from build123d import *

# Parameters (mm, degrees)
F1_DEPTH = 15
F4_D     = 4.1
F4_DEPTH = 7
F5_D     = 6.1
F5_DEPTH = 7


with BuildPart() as f1:
    # F0 (on Top) → F1 (new body)
    with BuildSketch(Plane.XY):
        Polygon((-8.678603, -7.1), (-8.678603, -5.1), (-10.678603, -7.1), (-10.678603, -13.5), (16.421397, -13.5), (16.421397, 13), (11.421397, 13), (11.421397, -7.1), (6.971397, -7.1), (6.971397, -10.4), (-4.228603, -10.4), (-4.228603, -7.1), align=None)
    extrude(amount=F1_DEPTH)

    # F4
    with Locations(Plane.YZ.offset(16.421397)):
        with Locations((3, 7.5)):
            Hole(F4_D / 2, depth=F4_DEPTH)

    # F5
    with Locations(Plane.XZ.offset(13.5)):
        with Locations((1.371397, 7.5)):
            Hole(F5_D / 2, depth=F5_DEPTH)


solid = f1.part
Could you check a few things on this model? Use its own coordinates, in mm. A direction names the side the tool comes from. Give positions to 0.01 mm unless a question says otherwise; leave off trailing zeros. Order: outer loops, then holes, each group sorted by start corner. A loop starts at its lowest first (then second) coordinate and runs counter-clockwise, first axis right, second up.
Item 1: I need wall thicknesses on line 1 (X direction, y = -7.75, z = 1); line 2 (Z direction, x = 15.05, y = 3); line 3 (Y direction, x = 7.75, z = 1). Which ranges of each line are inside material? Lowest first, please.
Item 2: If we section it at D-D, the plane z = 13: Write out the boundary of the cut face in (x, y).
Item 3: If we section it at B-B, the plane z = 7.5: Write out the boundary of the cut face in (x, y).
Item 4: I'm going to push flat-ended pins straight in: pin 1 (3.5 mm diameter, centred on y = 3, z = 7.5, fed in from -X); pin 2 (3.5 mm diameter, centred on x = 2.5, z = 6, fed in from +Y); pin 3 (1.3 mm diameter, centred on x = -6, z = 11, fed in from +Y). Where does each tip first touch, or does it pass through?
Item 5: If we section it at C-C, the plane x = 12.5: Write out the boundary of the cut face in (y, z), plus the area to 3 significant figures.
Item 6: If we mould it in two halves opening along Y, with no side actions, what happens to faces 3 (the face through (13.89, 1.11, 6.71)), 4 (the face through (-9.665, -6.086, 7.395)), 5 (the face through (-8.679, -6, 7))? For each: pulls with the +Y half, pulls with the -Y half, needs draft (parallel to the pull), parting line crosses it, or undercut.
Item 7: For faces 1 (the face through (-4.229, -9, 7)), 2 (the face through (16.421, 0, 7)), which set-ups out of +Z, -Z, +X, -X, +Y, -Y let a thin tool reach every point of the face, with its end or its side?
Item 8: If we section it at A-A, the plane y = 3: Write out the boundary of the cut face in (x, z), plus the area to 3 significant figures.
Values:
1. line 1: x = -10.68 to -4.23, 6.97 to 16.42
1. line 2: z = 0 to 5.45, 9.55 to 15
1. line 3: y = -13.5 to -7.1
2. outline: (-10.68, -13.5) - (16.42, -13.5) - (16.42, 13) - (11.42, 13) - (11.42, -7.1) - (6.97, -7.1) - (6.97, -10.4) - (-4.23, -10.4) - (-4.23, -7.1) - (-8.68, -7.1) - (-8.68, -5.1) - (-10.68, -7.1) - close
3. outline: (-10.68, -13.5) - (-1.68, -13.5) - (-1.68, -10.4) - (-4.23, -10.4) - (-4.23, -7.1) - (-8.68, -7.1) - (-8.68, -5.1) - (-10.68, -7.1) - close; (4.42, -13.5) - (16.42, -13.5) - (16.42, 0.95) - (11.42, 0.95) - (11.42, -7.1) - (6.97, -7.1) - (6.97, -10.4) - (4.42, -10.4) - close; (11.42, 5.05) - (16.42, 5.05) - (16.42, 13) - (11.42, 13) - close
4. pin 1: passes through
4. pin 2: stops at y = -10.4
4. pin 3: stops at y = -7.1
5. outline: (-13.5, 0) - (13, 0) - (13, 15) - (-13.5, 15) - close; hole circle Ø4.1 at (3, 7.5)
5. area: 384 mm2
6. face 3: undercut
6. face 4: pulls with the +Y half
6. face 5: needs draft
7. face 1: +Z, -Z, +Y
7. face 2: +Z, -Z, +X, +Y, -Y
8. outline: (11.42, 0) - (16.42, 0) - (16.42, 5.45) - (11.42, 5.45) - close; (11.42, 9.55) - (16.42, 9.55) - (16.42, 15) - (11.42, 15) - close
8. area: 54.5 mm2
